The drawing under review shows one solid part. Ordinate dimensions are in mm from its lowest x, y, z. Round coordinates to 2 decimals unless told otherwise and drop trailing zeros. Order: outer loops, then holes, each group sorted by start corner. A loop starts at its lowest first (then second) coordinate and runs counter-clockwise, first axis right, second up. Notation, with made-up numbers: M 76,-10 L 112,-10 A20 ccw 112,20 Z; hole C -40,40 d4. An arc over 180 degrees is marked long. Use a Markdown table: item, result.
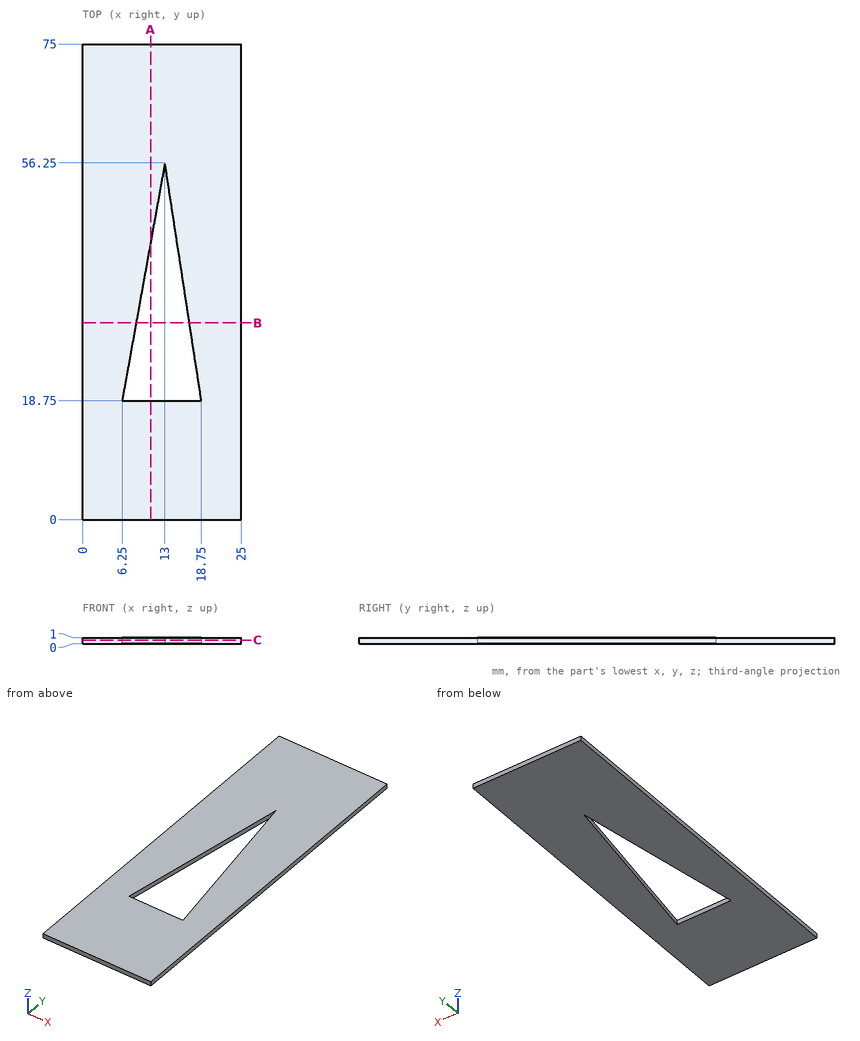
Q1. Add section B-B (y = 31). Write out the cut boundary in (x, z) (3 decimals), then the cut area to 3 significant figures.
Determined:
| item | result |
|---|---|
| outline | M 0,0 L 8.455,0 L 8.455,1 L 0,1 Z; M 16.872,0 L 25,0 L 25,1 L 16.872,1 Z |
| area | 16.6 mm^2 |
Q2. Add section C-C (z = 0.6). Write out the cut boundary in (x, y).
Determined:
| item | result |
|---|---|
| outline | M 0,0 L 25,0 L 25,75 L 0,75 Z; hole M 6.25,18.75 L 18.75,18.75 L 13,56.25 Z |
Q3. Clearance check with a flat-ended pin moving along its axis: pin 1 (5 mm diameter, centred on x = 13.5, y = 31.5, fed in from -Z). State where the tip first meets the part, or that it passes through.
Determined:
| item | result |
|---|---|
| pin 1 | passes through |
Q4. Wall thickness on line 1 along X through (y, z) = (39.5, 0.55) (3 decimals); line 2 along X through (y, z) = (28, 0.2) (3 decimals): over which ranges is each line inside the solid? List them lowest first. Write a range as [from, to].
Determined:
| item | result |
|---|---|
| line 1 | x = [0, 9.985], [15.568, 25] |
| line 2 | x = [0, 7.915], [17.332, 25] |
Q5. Add section A-A (x = 10.75). Write out the cut boundary in (y, z).
Determined:
| item | result |
|---|---|
| outline | M 0,0 L 18.75,0 L 18.75,1 L 0,1 Z; M 43.75,0 L 75,0 L 75,1 L 43.75,1 Z |
